from build123d import *

# Parameters (mm, degrees)
F0_W     = 90
F0_H     = 118
F1_DEPTH = 6
F2_W     = 90
F2_H     = 50
F3_DEPTH = 6
F4_W     = 5.5
F4_H     = 10
F5_DEPTH = 6
F6_W     = 15
F6_H     = 5.5
F7_DEPTH = 6


with BuildPart() as f1:
    # F0 (on Top) → F1 (new body)
    with BuildSketch(Plane.XY):
        Rectangle(F0_W, F0_H)
    extrude(amount=F1_DEPTH)

    # F2 (on face) → F3 (join)
    with BuildSketch(Plane.XY.offset(6)):
        with Locations((0, 84)):
            Rectangle(F2_W, F2_H)
    extrude(amount=-F3_DEPTH)

    # F4 (on face) → F5 (cut)
    with BuildSketch(Plane.XY.offset(6)):
        with Locations((-37.5, 50)):
            Rectangle(F4_W, F4_H)
        with Locations((37.5, 50)):
            Rectangle(F4_W, F4_H)
        with Locations((37.5, -50)):
            Rectangle(F4_W, F4_H)
        with Locations((-37.5, -50)):
            Rectangle(F4_W, F4_H)
    extrude(amount=-F5_DEPTH, mode=Mode.SUBTRACT)

    # F6 (on face) → F7 (cut)
    with BuildSketch(Plane.XY.offset(6)):
        with Locations((-32.5, 61.25)):
            Rectangle(F6_W, F6_H)
        with Locations((32.5, 61.25)):
            Rectangle(F6_W, F6_H)
        with Locations((-32.5, 87.582247)):
            Rectangle(F6_W, F6_H)
        with Locations((32.5, 87.582247)):
            Rectangle(F6_W, F6_H)
    extrude(amount=-F7_DEPTH, mode=Mode.SUBTRACT)


solid = f1.part
For this review, take the finished solid that the model builds, in its own axes (mm). A direction names the side the tool comes from. Round coordinates to 2 decimals unless told otherwise and drop trailing zeros. Write each loop counter-clockwise with the first axis right and the second up, starting at its lowest first coordinate (ties: lowest second). Pieces come first, ordered by that corner, then holes. Notation, with made-up numbers: (-18.75, -21.75) - (-11.75, -21.75) arc R26 cw to (-11.75, 1.25) - close; hole circle Ø7 at (-9.75, 65). An arc over 180 degrees is marked (long way). Write item = value, one per line. Start each with the question number.
1. Consider section B-B on z = 3.85. Give the number of separate pieces and of enclosed holes in the cut face, plus the area to 3 significant figures.
2. For faces 4 (the face through (25, 61, 3)), 5 (the face through (45, 24, 3)), list the 3-axis set-ups (+Z, -Z, +X, -X, +Y, -Y) from which the entire face can be reached by the end or side of a thin tool; tool diameter is ignored.
3. Consider section A-A on x = -30.5. State the section outline as (y, z) points, plus the area to 3 significant figures.
4. Draft analysis for pull direction Y (two halves, no side actions). For faces 1 (the face through (-1, -59, 3)), 2 (the face through (-1, 26, 6)), 3 (the face through (-38, 45, 3)), state which applies: released by +Y, released by -Y, zero draft, split by the parting line, or undercut.
5. Wall thickness on L1, parallel to Y at x = 35.5, z = 4.1; L2, parallel to Y at x = 33, z = 5.15; L3, parallel to X at y = -47, z = 5.2: over which ranges is each line inside the solid? List them lowest first.
Evaluation:
q1.separate_pieces = 1
q1.enclosed_holes = 8
q1.area = 14,600 mm2
q2.face_4 = +Z, -Z
q2.face_5 = +Z, -Z, +X, +Y, -Y
q3.outline = (-59, 0) - (58.5, 0) - (58.5, 6) - (-59, 6) - close; (64, 0) - (84.83, 0) - (84.83, 6) - (64, 6) - close; (90.33, 0) - (109, 0) - (109, 6) - (90.33, 6) - close
q3.area = 942 mm2
q4.face_1 = released by -Y
q4.face_2 = zero draft
q4.face_3 = undercut
q5.L1 = -59 to -55, -45 to 45, 55 to 58.5, 64 to 84.83, 90.33 to 109
q5.L2 = -59 to 58.5, 64 to 84.83, 90.33 to 109
q5.L3 = -45 to -40.25, -34.75 to 34.75, 40.25 to 45
